Read the model definition and answer for the solid it produces. Units are mm, in the model's axes. Coordinates: 2 decimals unless noted, no trailing zeros. Write each loop counter-clockwise with the first axis right and the second up, starting at its lowest first coordinate (ties: lowest second). Pieces come first, ordered by that corner, then holes.
(1) Section A-A on x = 0 is taken. Write down the section's boundary in (y, z), then the cut area to 3 significant figures.
(2) Find the intervals of material crossed by probe 1 along X at (y, z) = (3.35, 0); probe 2 along Z at (x, y) = (7, 5.1); probe 3 along X at (y, z) = (0.45, -15), in increasing order.
(3) Section C-C on y = 4.45 is taken. Write down the section's boundary in (x, z).
(4) The mould has two halves that part along Z. Classify faces 1 (the flat face through (0, 3, 20)), 2 (the flat face through (0, 3, -20)), 3 (the cylindrical face through (7.3, 3, -13.8)): +Z half, -Z half, draft (parallel to the pull), parting line (faces both ways), or undercut.
(5) Section B-B on z = 0 is taken. Write down the section's boundary in (x, y).
from build123d import *

# Parameters (mm, degrees)
SKETCH1_W           = 60
SKETCH1_H           = 40
SKETCH1_R           = 4
BOSS_EXTRUDE1_DEPTH = 6
SKETCH2_R           = 1.65
CUT_EXTRUDE1_DEPTH  = 10


with BuildPart() as part:
    # Sketch1 → Boss-Extrude1 (new body)
    with BuildSketch(Plane(origin=(0, 0, 0), x_dir=(1, 0, 0), z_dir=(0, 1, 0))):
        Rectangle(SKETCH1_W, SKETCH1_H)
        with Locations(Location((0, 0, 0), (0, 0, 270))):
            Circle(SKETCH1_R, mode=Mode.SUBTRACT)
    extrude(amount=BOSS_EXTRUDE1_DEPTH)

    # Sketch2 → Cut-Extrude1 (cut)
    with BuildSketch(Plane(origin=(0, 6, 0), x_dir=(1, 0, 0), z_dir=(0, 1, 0))):
        with Locations(Location((6.795088799, 15.372923216, 0), (0, 0, 270))):
            Circle(SKETCH2_R)
        with Locations(Location((6.202536092, -15.621413061, 0), (0, 0, 270))):
            Circle(SKETCH2_R)
    extrude(amount=-CUT_EXTRUDE1_DEPTH, mode=Mode.SUBTRACT)


solid = part.part
Response:
1. outline: (0, -20) - (6, -20) - (6, -4) - (0, -4) - close; (0, 4) - (6, 4) - (6, 20) - (0, 20) - close
1. area: 192 mm2
2. probe 1: x = -30 to -4, 4 to 30
2. probe 2: z = -20 to -17.01, -13.74 to 14.18, 17.07 to 20
2. probe 3: x = -30 to 5.19, 8.4 to 30
3. outline: (-30, -20) - (30, -20) - (30, 20) - (-30, 20) - close; hole circle Ø8 at (0, 0); hole circle Ø3.3 at (6.2, 15.62); hole circle Ø3.3 at (6.8, -15.37)
4. face 1: +Z half
4. face 2: -Z half
4. face 3: undercut
5. outline: (-30, 0) - (-4, 0) - (-4, 6) - (-30, 6) - close; (4, 0) - (30, 0) - (30, 6) - (4, 6) - close
